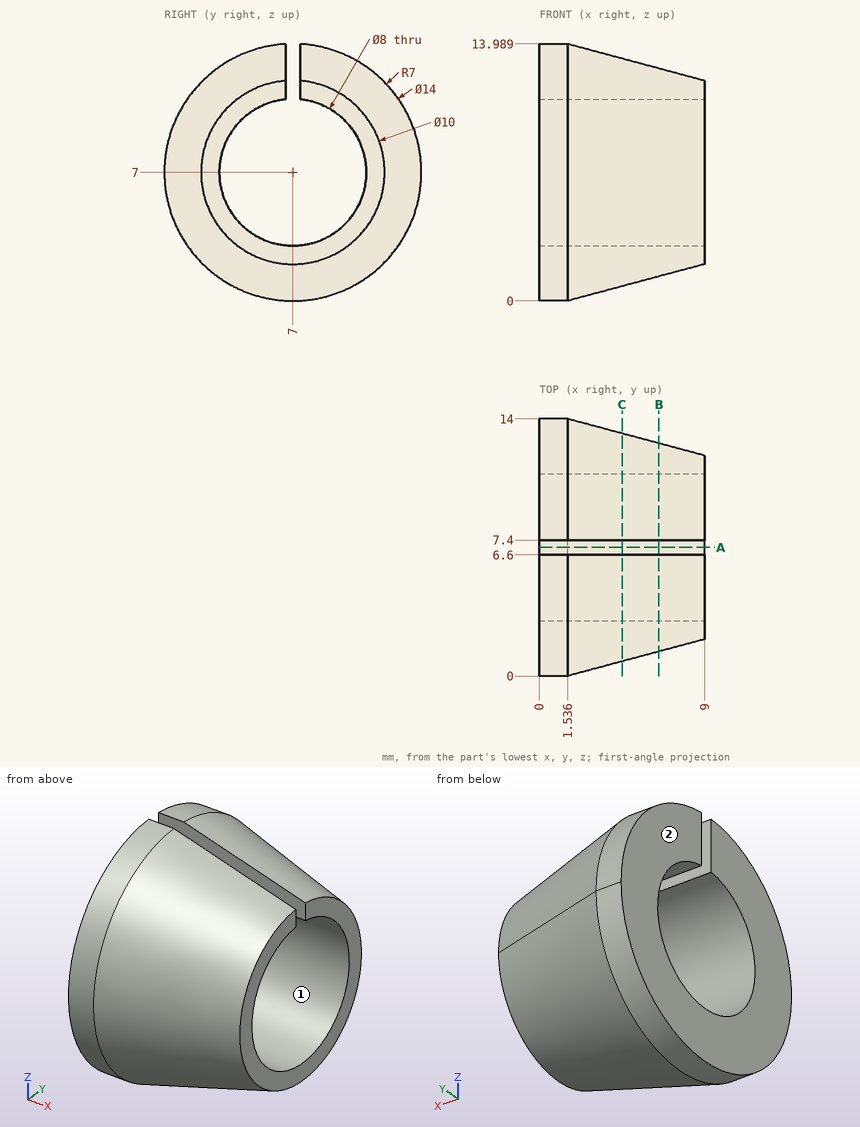
Here's the drawing with two shaded views (mm, measured from the low corner). I have some questions. Give positions to 0.01 mm unless a question says otherwise; leave off trailing zeros. Write each loop counter-clockwise with the first axis right and the second up, starting at its lowest first coordinate (ties: lowest second). Pieces come first, ordered by that corner, then holes. Notation, with made-up numbers: (42, 18.25) -> (94, 18.25) arc R26 cw to (94, 35.25) -> close; hole circle Ø3 at (19.25, 83). An arc over 180 degrees is marked (long way). One line per item, written item: value.
Q1. Imagine slicing it at C-C on x = 4.5. Please give me the cut outline in (y, z) (1 decimal).
Results found:
outline: (6.6, 11) -> (6.6, 13.2) arc R6.2 ccw (long way) to (7.4, 13.2) -> (7.4, 11) arc R4 cw (long way) to start
Q2. Imagine slicing it at A-A on y = 7. Please give me the cut outline in (x, z).
Results found:
outline: (0, 0) -> (1.54, 0) -> (9, 2) -> (9, 3) -> (0, 3) -> close
Q3. Please list where these lines run through material, in increasing order: line 1 (Y direction, x = 2.5, z = 9) (1 decimal); line 2 (Y direction, x = 3.75, z = 7); line 3 (Z direction, x = 5.5, y = 7.5). Write a range as [from, to].
Results found:
line 1: y = [0.6, 3.5], [10.5, 13.4]
line 2: y = [0.59, 3], [11, 13.41]
line 3: z = [1.08, 3.03], [10.97, 12.92]
Q4. Imagine slicing it at B-B on x = 6.5. Please give me the cut outline in (y, z) (1 decimal).
Results found:
outline: (6.6, 11) -> (6.6, 12.7) arc R5.7 ccw (long way) to (7.4, 12.7) -> (7.4, 11) arc R4 cw (long way) to start
Q5. For P1, Ø3.5, axis at x = 5.5, z = 12.5, coming from the -Y side; P2, Ø3.5, axis at x = 4, z = 13, coming from the +Y side (1 decimal); P3, Ø3, axis at x = 4, y = 9, coming from the -Z side, each with a flat end and sliding along its axis, tell me the tip position at first contact or that it passes through.
Results found:
P1: stops at y = 2.27
P2: stops at y = 11.8
P3: stops at z = 0.43
Q6. We'd pull the mould along Y, two halves only. Please class the marked faces 1 and 2: +Y half, -Y half, draft (parallel to the pull), parting line (faces both ways), or undercut.
Results found:
face 1: undercut
face 2: draft
